from build123d import *

# Parameters (mm, degrees)
EXTRUDE1_DEPTH = 5
EXTRUDE2_DEPTH = 50
SKETCH3_R      = 4.7625
EXTRUDE3_DEPTH = 101.763138101
EXTRUDE4_REACH = 106.149
SKETCH4_R      = 4.7625
EXTRUDE5_REACH = 106.149
SKETCH5_R      = 4.7625


with BuildPart() as part:
    # Sketch1 → Extrude1 (new body)
    with BuildSketch(Plane.XY):
        Polygon((0, 9.929325872), (58.847804665, 0), (88.9, 0), (0, 15), align=None)
        Polygon((0, 9.929325872), (0, 0), (58.847804665, 0), align=None)
        Polygon((58.847804665, 0), (0, 0), (0, -9.929325872), align=None)
        Polygon((88.9, 0), (58.847804665, 0), (0, -9.929325872), (0, -15), align=None)
    extrude(amount=EXTRUDE1_DEPTH)

    # Sketch1_4 → Extrude2 (add)
    with BuildSketch(Plane.XY):
        Polygon((0, 9.929325872), (58.847804665, 0), (88.9, 0), (0, 15), align=None)
        Polygon((88.9, 0), (58.847804665, 0), (0, -9.929325872), (0, -15), align=None)
    extrude(amount=EXTRUDE2_DEPTH)

    # Sketch3 → Extrude3 (cut, through all)
    with BuildSketch(Plane.XY.offset(5)):
        with Locations((12.7, 0)):
            Circle(SKETCH3_R)
    extrude(amount=-EXTRUDE3_DEPTH, mode=Mode.SUBTRACT)

    # Sketch4 → Extrude4 (cut, up to next)
    with BuildSketch(Plane(origin=(2.460873919, -14.584779429, 0), x_dir=(0.9860621829168484, 0.16637719621769093, 0), z_dir=(0.16637719621769093, -0.9860621829168484, 0)), mode=Mode.PRIVATE) as extrude4_sk1:
        with Locations((10.204342057, 25)):
            Circle(SKETCH4_R)
    extrude4_tool1 = extrude(extrude4_sk1.sketch, amount=-EXTRUDE4_REACH, mode=Mode.PRIVATE) & part.part
    add(extrude4_tool1.solids().sort_by_distance((12.52299, -12.88701, 25))[0], mode=Mode.SUBTRACT)

    # Sketch5 → Extrude5 (cut, up to next)
    with BuildSketch(Plane(origin=(2.460873919, 14.584779429, 0), x_dir=(0.9860621829168484, -0.16637719621769093, 0), z_dir=(0.16637719621769093, 0.9860621829168484, 0)), mode=Mode.PRIVATE) as extrude5_sk1:
        with Locations(Location((10.204342057, -25, 0), (0, 0, 180))):
            Circle(SKETCH5_R)
    extrude5_tool1 = extrude(extrude5_sk1.sketch, amount=-EXTRUDE5_REACH, mode=Mode.PRIVATE) & part.part
    add(extrude5_tool1.solids().sort_by_distance((12.52299, 12.88701, 25))[0], mode=Mode.SUBTRACT)


solid = part.part
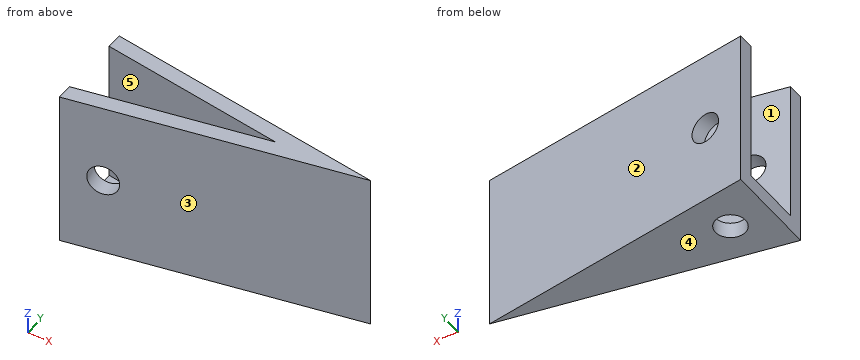
Design review of the part built by this model. Coordinates are the model's own, in mm. Face numbers are marked on the shaded views. A direction names the side the tool comes from. Round coordinates to 2 decimals unless told otherwise and drop trailing zeros. Write each loop counter-clockwise with the first axis right and the second up, starting at its lowest first coordinate (ties: lowest second). Pieces come first, ordered by that corner, then holes. Notation, with made-up numbers: (-31.75, 32.5) - (-26.75, 32.5) arc R23 cw to (-26.75, 58.5) - close; hole circle Ø11 at (-31, 34.5). An arc over 180 degrees is marked (long way). Use a Markdown table: item, result. Add a question column.
1. Wall thickness on probe 1 along Y at (x, z) = (17, 21.5); probe 2 along Z at (x, y) = (13.5, -6); probe 3 along Y at (x, z) = (56, 11): over which ranges is each line inside the solid? List them lowest first.
2. For the marked faces 1 and 2, list the 3-axis set-ups (+Z, -Z, +X, -X, +Y, -Y) from which the entire face can be reached by the end or side of a thin tool; tool diameter is ignored.
3. We need section A-A (z = 22.5). State the section outline as (x, y) points.
4. We need section C-C (z = 16.5). State the section outline as (x, y) points.
5. We need section B-B (x = 31). State the section outline as (y, z) points, then the cut area to 3 significant figures.
6. We need section D-D (x = 12.7). Count the separate pieces of the cut face and the enclosed holes in it, then the cut area to 3 significant figures.
7. Clearance check with flat-ended pins moving along their axes: pin 1 (1 mm diameter, centred on x = 45.5, z = 12, fed in from +Y); pin 2 (1.5 mm diameter, centred on x = 48.5, z = 25.5, fed in from +Y); pin 3 (3 mm diameter, centred on x = 65, z = 35, fed in from +Y). State where each tip first meets the part, or that it passes through.
8. Mouldability with a two-part tool opening along Y and no side actions: class the marked faces 3, 4 and 5 as +Y half, -Y half, draft (parallel to the pull), parting line (faces both ways), or undercut.
Output:
| question | item | result |
|---|---|---|
| 1 | probe 1 | y = -12.13 to -7.06, 7.06 to 12.13 |
| 1 | probe 2 | z = 0 to 5 |
| 1 | probe 3 | y = -5.55 to -0.48, 0.48 to 5.55 |
| 2 | face 1 | +Z, -X |
| 2 | face 2 | +Z, -Z, +X, +Y |
| 3 | outline | (0, -15) - (8.53, -13.56) - (7.69, -8.63) - (0, -9.93) - close; (0, 9.93) - (7.69, 8.63) - (8.53, 13.56) - (0, 15) - close; (15.69, -7.28) - (16.52, -12.21) - (88.9, 0) - (16.52, 12.21) - (15.69, 7.28) - (58.85, 0) - close |
| 4 | outline | (0, -15) - (88.9, 0) - (0, 15) - (0, 9.93) - (58.85, 0) - (0, -9.93) - close |
| 5 | outline | (-9.77, 0) - (9.77, 0) - (9.77, 50) - (4.7, 50) - (4.7, 5) - (-4.7, 5) - (-4.7, 50) - (-9.77, 50) - close |
| 5 | area | 554 mm2 |
| 6 | separate pieces | 4 |
| 6 | enclosed holes | 0 |
| 6 | area | 442 mm2 |
| 7 | pin 1 | stops at y = 7.41 |
| 7 | pin 2 | stops at y = 6.94 |
| 7 | pin 3 | stops at y = 4.29 |
| 8 | face 3 | -Y half |
| 8 | face 4 | draft |
| 8 | face 5 | undercut |
